Can you work these out from the model? Positions are in its coordinate system, mm. A direction names the side the tool comes from. Give positions to 0.01 mm unless a question says otherwise; leave off trailing zeros. Write each loop counter-clockwise with the first axis right and the second up, starting at its lowest first coordinate (ties: lowest second). Pieces come first, ordered by that corner, then holes. Notation, with made-up numbers: M -2.5,-33 L 42.5,-33 A23 cw 42.5,-8 Z; hole C -29,64 d10. An arc over 180 degrees is marked long. Write each question's results on one line, items separated by ' | '.
Autodesk Inventor part; units mm, degrees
ref_plane "YZ Plane" through (0, 0, 0) normal (1, 0, 0) x (0, 1, 0)
ref_plane "XZ Plane" through (0, 0, 0) normal (0, 1, 0) x (-1, 0, 0)
ref_plane "XY Plane" through (0, 0, 0) normal (0, 0, 1) x (1, 0, 0)
sketch "Profile" plane through (0, 0, 0) normal (0, 0, 1) x (1, 0, 0)
  line L0 (-24, 0) -> (-24, 11)
  line L1 (-24, 11) -> (0, 11)
  line L2 (0, 11) -> (0.5774, 12)
  line L3 (0.5774, 12) -> (50.5774, 12)
  line L4 (50.5774, 12) -> (51.1547, 11)
  line L5 (51.1547, 11) -> (76, 11)
  line L6 (76, 11) -> (76, 0)
  line L7 (-24, 0) -> (0, 0)
  line L8 (0, 0) -> (0, 9)
  line L9 (0, 9) -> (68, 9)
  line L10 (68, 9) -> (68, 0)
  line L11 (68, 0) -> (76, 0)
  line L12 (-44, 0) -> (96, 0) construction
  line L13 (0, 11) -> (0, 9) construction
  dimension "BodyLength" = 100
  dimension "d1" = 11
  dimension "d3" = 120
  dimension "d4" = 120
  dimension "d5" = 50
  dimension "d6" = 24
  dimension "d16" = 8
  dimension "d29" = 1
  dimension "d30" = 9
revolve "ProfileRevolveFeature" add sketch "Profile" angle 360 about axis through (-10, 0, 0) along (1, 0, 0)
sketch "InsideHole" plane through (-24, 0, 0) normal (-1, 0, 0) x (0, 0, 1)
  circle A0 centre (0, 0) radius 9 construction
hole "InsideHoleFeature" at (-24, 0, 0) direction (1, 0, 0) diameter 19 end through all
chamfer "EndChamferFeature" distance 1 angle 45 1 edges at (-24, -11, 0)
sketch "CapMountHole" plane through (0, 0, 0) normal (0, 1, 0) x (-1, 0, 0)
  line L0 (-76, 11) -> (-76, -11) construction
  line L1 (9.12, 0) -> (-54.72, 0) construction
  circle A0 centre (-71.5, 0) radius 1.25
  point P0 (0, 0)
  dimension "d31" = 4.5
  dimension "d39" = 2.5
extrude "CapMountHoleFeature" cut sketch "CapMountHole" along normal through all both and the other way through all
equation "\"d5\" = 0.5 * BodyLength"
equation "\"d6\" = 0.24 * BodyLength"
properties part number "BackPair1PistonBody"
Item 1: I want a section at B-B, the plane y = 0. Please give me the cut outline in (x, z), and give its area (3 significant figures).
Geometry says:
outline: M -24,-10 L -23,-11 L 0,-11 L 0.58,-12 L 50.58,-12 L 51.15,-11 L 76,-11 L 76,-9.5 L -24,-9.5 Z; M -24,9.5 L 76,9.5 L 76,11 L 51.15,11 L 50.58,12 L 0.58,12 L 0,11 L -23,11 L -24,10 Z | area: 400 mm2
Item 2: I want a section at A-A, the plane z = 0. Please give me the cut outline in (x, y), and give its area (3 significant figures).
Geometry says:
outline: M -24,-10 L -23,-11 L 0,-11 L 0.58,-12 L 50.58,-12 L 51.15,-11 L 70.25,-11 L 70.25,-9.5 L -24,-9.5 Z; M -24,9.5 L 70.25,9.5 L 70.25,11 L 51.15,11 L 50.58,12 L 0.58,12 L 0,11 L -23,11 L -24,10 Z; M 72.75,-11 L 76,-11 L 76,-9.5 L 72.75,-9.5 Z; M 72.75,9.5 L 76,9.5 L 76,11 L 72.75,11 Z | area: 393 mm2
Item 3: For faces 4 (the face through (-11.34, -2.38, -10.74)), 5 (the face through (-24, 9, -4)), 6 (the face through (63.751, 10.161, -4.213)), which set-ups out of +Z, -Z, +X, -X, +Y, -Y let a thin tool reach every point of the face, with its end or its side?
Geometry says:
face 4: -X | face 5: +Z, -Z, -X, +Y, -Y | face 6: +X
Item 4: If I drill on line 1 (Y direction, x = -8.5, z = -0.5); line 2 (Z direction, x = 44.5, y = -1.75); line 3 (Z direction, x = 42, y = -8.5), over which ranges is the centre line in solid material (lowest first)? Write a range as from..to.
Geometry says:
line 1: y = -10.99..-9.49, 9.49..10.99 | line 2: z = -11.87..-9.34, 9.34..11.87 | line 3: z = -8.47..-4.24, 4.24..8.47
Item 5: Thinking about a two-plate mould opening in Z: for faces 1 (the face through (26.7, 8.43, 4.38)), 2 (the face through (76, -10, 0)), 3 (the face through (25.93, -11.99, 0.53)), which applies, +Z half, -Z half, draft (parallel to the pull), parting line (faces both ways), or undercut?
Geometry says:
face 1: undercut | face 2: draft | face 3: parting line
Item 6: I want a section at D-D, the plane x = -9.5. Please give me the cut outline in (y, z), and give its area (3 significant figures).
Geometry says:
outline: C 0,0 d22; hole C 0,0 d19 | area: 96.6 mm2
Item 7: I'm going to push flat-ended pins straight in: pin 1 (2 mm diameter, centred on y = -7.5, z = 5.5, fed in from +X); pin 2 (1.5 mm diameter, centred on x = 71.5, z = 0, fed in from -Y); pin 3 (2 mm diameter, centred on x = 20.5, z = -2, fed in from -Y); pin 4 (3 mm diameter, centred on x = 71.5, z = 0, fed in from -Y). Where does each tip first touch, or does it pass through?
Geometry says:
pin 1: stops at x = 76 | pin 2: passes through | pin 3: stops at y = -11.96 | pin 4: stops at y = -11
Item 8: I want a section at C-C, the plane x = 71.5. Please give me the cut outline in (y, z), and give its area (3 significant figures).
Geometry says:
outline: M -10.93,-1.25 A11 ccw 10.93,-1.25 L 9.42,-1.25 A9.5 cw -9.42,-1.25 Z; M -10.93,1.25 L -9.42,1.25 A9.5 cw 9.42,1.25 L 10.93,1.25 A11 ccw Z | area: 89.1 mm2
